For this review, take the finished solid that the model builds, in its own axes (mm). Face numbers are marked on the shaded views. A direction names the side the tool comes from. Give positions to 0.01 mm unless a question says otherwise; leave off trailing zeros. Loops run counter-clockwise (first coordinate to the right, second up) from the corner with the lowest first, then second, coordinate; pieces in that order, holes last.
```python
from build123d import *

# Parameters (mm, degrees)
ESQUISSE1_R                      = 12.05
ESQUISSE1_R_2                    = 10.05
BASE_DEPTH                       = 10
BOSS_TIGE_DEPTH                  = 2
CONGE_TIGE_R                     = 0.2
REP_SUPPORT_TIGE_COUNT           = 5
CONGE_TIGE_OF_REP_SUPPORT_TIGE_R = 0.2


with BuildPart() as part:
    # Esquisse1 → BASE (new body)
    with BuildSketch(Plane(origin=(0, 0, 0), x_dir=(1, 0, 0), z_dir=(0, 1, 0))):
        with Locations(Location((0, 0, 0), (0, 0, 270))):
            Circle(ESQUISSE1_R)
        with Locations(Location((0, 0, 0), (0, 0, 270))):
            Circle(ESQUISSE1_R_2, mode=Mode.SUBTRACT)
    extrude(amount=BASE_DEPTH)

    # Esquisse7 → BOSS TIGE (add)
    with BuildSketch(Plane(origin=(0, 0, 2.6), x_dir=(-1, 0, 0), z_dir=(0, 0, -1))):
        with BuildLine():
            Line((14.022631891, 9.608391049), (11.415742159, 9.608391049))
            Line((11.415742159, 9.608391049), (11.415742159, 4.685414017))
            Line((11.415742159, 4.685414017), (18.629521623, 4.685414017))
            Line((18.629521623, 4.685414017), (18.629521623, 9.608391049))
            Line((18.629521623, 9.608391049), (16.022631891, 9.608391049))
            Line((16.022631891, 9.608391049), (16.302913172, 8.020618644))
            ThreePointArc((16.302913172, 8.020618644), (15.022631891, 5.596902533), (13.742350611, 8.020618644))
            Line((13.742350611, 8.020618644), (14.022631891, 9.608391049))
        make_face()
    boss_tige = extrude(amount=BOSS_TIGE_DEPTH)

    # CONGE TIGE
    conge_tige_edges = [part.edges().sort_by_distance(p)[0] for p in [
        (-14.022631891, 9.608391049, 1.6),
        (-16.022631891, 9.608391049, 1.6),
    ]]
    fillet(conge_tige_edges, radius=CONGE_TIGE_R)

    # REP SUPPORT TIGE: BOSS TIGE ×5 about axis
    rep_support_tige_axis = Axis((0, 0, 0), (0, 1, 0))
    for i in range(1, REP_SUPPORT_TIGE_COUNT):
        add(boss_tige.rotate(rep_support_tige_axis, i * 360 / REP_SUPPORT_TIGE_COUNT))

    # CONGE TIGE of REP SUPPORT TIGE
    conge_tige_of_rep_support_tige_edges = [part.edges().sort_by_distance(p)[0] for p in [
        (-2.811541134, 9.608391049, 13.830742627),
        (-3.429575123, 9.608391049, 15.732855659),
        (12.285003909, 9.608391049, 6.947869033),
        (13.903037898, 9.608391049, 8.123439537),
        (10.404091102, 9.608391049, -9.536723415),
        (12.022125091, 9.608391049, -10.712293919),
        (-5.854921986, 9.608391049, -12.841888245),
        (-6.472955975, 9.608391049, -14.744001277),
    ]]
    fillet(conge_tige_of_rep_support_tige_edges, radius=CONGE_TIGE_OF_REP_SUPPORT_TIGE_R)


solid = part.part
```
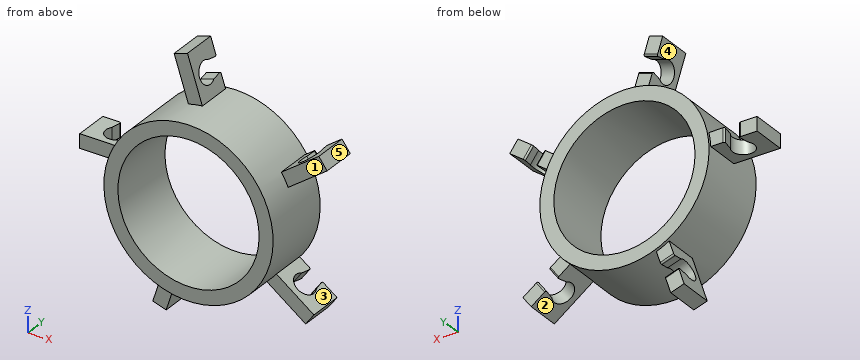
Q1. Mouldability with a two-part tool opening along X and no side actions: class the marked faces 1, 2 and 3 as +X half, -X half, draft (parallel to the pull), parting line (faces both ways), or undercut.
Answers:
face 1: draft
face 2: undercut
face 3: +X half
Q2. Consider section A-A on x = 0. Give the boundary of the cut face in (y, z).
Answers:
outline: (0, -12.05) - (10, -12.05) - (10, -10.05) - (0, -10.05) - close; (0, 10.05) - (10, 10.05) - (10, 12.05) - (0, 12.05) - close
Q3. For probe 1 along Y at (x, z) = (13, -11.5); probe 2 along X at (y, z) = (0.5, -5); probe 3 along Z at (x, y) = (6, 9.25), list the stretches that pass through material, from the lowest coordinate up.
Answers:
probe 1: y = 4.69 to 9.61
probe 2: x = -10.96 to -8.72, 8.72 to 10.96
probe 3: z = -10.45 to -8.06, 8.06 to 10.45
Q4. Consider section B-B on z = 0. Give the boundary of the cut face in (x, y), plus the area to 3 significant figures.
Answers:
outline: (-12.05, 0) - (-10.05, 0) - (-10.05, 10) - (-12.05, 10) - close; (10.05, 0) - (12.05, 0) - (12.05, 10) - (10.05, 10) - close
area: 40.0 mm2
Q5. Consider section C-C on y = 8.5. Count the separate pieces of the cut face and the enclosed holes in it, plus the area to 3 significant figures.
Answers:
separate pieces: 6
enclosed holes: 1
area: 182 mm2
Q6. Consider section D-D on y = 1.5. Give the boundary of the cut face in (x, z), plus the area to 3 significant figures.
Answers:
outline: circle Ø24.1 at (0, 0); hole circle Ø20.1 at (0, 0)
area: 139 mm2
Q7. Machinability: for the marked faces 4 and 5, which of the approach directions +Z, -Z, +X, -X, +Y, -Y give a long, thin tool a straight path to every point of the face, cutting with its end or side? Answer none if there is none.
Answers:
face 4: -X, +Y, -Y
face 5: +Z, +X, +Y, -Y
Q8. For pin 1 Ø1.3 at (x, z) = (-4, 17.5) entering from +Y; pin 2 Ø6 at (y, z) = (6.5, -5) entering from +X; pin 3 Ø3 at (y, z) = (1, -1) entering from -X; pin 4 Ø1.9 at (x, y) = (-15.02, 7.15) entering from +Z, all flat-tipped, find the tip position at first contact; note any pin that passes through.
Answers:
pin 1: stops at y = 9.61
pin 2: stops at x = 11.88
pin 3: stops at x = -12.05
pin 4: passes through
